Could you check a few things on this model? Use its own coordinates, in mm. A direction names the side the tool comes from. Coordinates: 2 decimals unless noted, no trailing zeros. Loops run counter-clockwise (first coordinate to the right, second up) from the corner with the lowest first, then second, coordinate; pieces in that order, holes last.
from build123d import *

# Parameters (mm, degrees)
SKETCH1_W                     = 42
SKETCH1_H                     = 20
BOSS_EXTRUDE1_DEPTH           = 40
CBORE_FOR_M5_SHCS1_AT_2_COUNT = 2
CBORE_FOR_M5_SHCS1_AT_2_PITCH = 20
SKETCH5_W                     = 42
SKETCH5_H                     = 20
BOSS_EXTRUDE2_DEPTH           = 6.5
SKETCH12_W                    = 21.9
SKETCH12_H                    = 10
BOSS_EXTRUDE3_DEPTH           = 46.5
CUT_EXTRUDE1_DEPTH            = 7.5
FILLET1_R                     = 1
CBORE_FOR_M3_SHCS2_AT_2_COUNT = 2
CBORE_FOR_M3_SHCS2_AT_2_PITCH = 20
CUT_EXTRUDE2_DEPTH            = 8


with BuildPart() as part:
    # Sketch1 → Boss-Extrude1 (new body)
    with BuildSketch(Plane(origin=(0, 0, 0), x_dir=(1, 0, 0), z_dir=(0, 1, 0))):
        Rectangle(SKETCH1_W, SKETCH1_H)
    extrude(amount=BOSS_EXTRUDE1_DEPTH)

    # Sketch4 → CBORE for M5 SHCS1 (revolve, cut)
    with BuildSketch(Plane(origin=(11, 30, 10), x_dir=(0, -1, 0), z_dir=(1, 0, 0))):
        Polygon((0, 0), (0, 20), (2.75, 20), (2.75, 5), (5, 5), (5, 0.020977491), (5.025, 0), align=None)
    cbore_for_m5_shcs1 = revolve(axis=Axis((11, 30, 16.35), (0, 0, -1)), mode=Mode.SUBTRACT)

    # CBORE for M5 SHCS1 at 2: CBORE for M5 SHCS1 ×2
    with Locations(*[(0, -i * CBORE_FOR_M5_SHCS1_AT_2_PITCH, 0) for i in range(1, CBORE_FOR_M5_SHCS1_AT_2_COUNT)]):
        add(cbore_for_m5_shcs1, mode=Mode.SUBTRACT)

    # Sketch5 → Boss-Extrude2 (add)
    with BuildSketch(Plane(origin=(0, 40, 0), x_dir=(1, 0, 0), z_dir=(0, 1, 0))):
        Rectangle(SKETCH5_W, SKETCH5_H)
    extrude(amount=BOSS_EXTRUDE2_DEPTH)

    # Sketch12 → Boss-Extrude3 (add)
    with BuildSketch(Plane(origin=(0, 46.5, 0), x_dir=(1, 0, 0), z_dir=(0, 1, 0))):
        with Locations((-10.05, 15)):
            Rectangle(SKETCH12_W, SKETCH12_H)
    extrude(amount=-BOSS_EXTRUDE3_DEPTH)

    # Sketch6 → Cut-Extrude1 (cut)
    with BuildSketch(Plane(origin=(0, 46.5, 0), x_dir=(1, 0, 0), z_dir=(0, 1, 0))):
        Polygon((-16.51, 20), (-16.51, -5), (-8.05, -5), (-8.05, 16), (-14.71, 16), (-14.71, 20), align=None)
    extrude(amount=-CUT_EXTRUDE1_DEPTH, mode=Mode.SUBTRACT)

    # Fillet1
    fillet1_edges = [part.edges().sort_by_distance(p)[0] for p in [
        (0.9, 23.25, -20),
        (-21, 23.25, -20),
        (21, 23.25, -10),
        (21, 23.25, 10),
        (-21, 23.25, 10),
    ]]
    fillet(fillet1_edges, radius=FILLET1_R)

    # Sketch11 → CBORE for M3 SHCS1 (revolve, cut)
    with BuildSketch(Plane(origin=(-11.48, 42.5, 10), x_dir=(0, -1, 0), z_dir=(1, 0, 0))):
        Polygon((0, 0), (0, 6.021463052), (1.7, 5), (1.7, 3), (3.25, 3), (3.25, 0.020977491), (3.275, 0), align=None)
    revolve(axis=Axis((-11.48, 42.5, 16.35), (0, 0, -1)), mode=Mode.SUBTRACT)

    # Sketch16 → CBORE for M3 SHCS2 (revolve, cut)
    with BuildSketch(Plane(origin=(-3.575, 46.5, -15), x_dir=(0, 0, 1), z_dir=(1, 0, 0))):
        Polygon((0, 0), (0, 46.5), (1.7, 46.5), (1.7, 3), (3.25, 3), (3.25, 0.020977491), (3.275, 0), align=None)
    cbore_for_m3_shcs2 = revolve(axis=Axis((-3.575, 52.85, -15), (0, -1, 0)), mode=Mode.SUBTRACT)

    # CBORE for M3 SHCS2 at 2: CBORE for M3 SHCS2 ×2
    with Locations(*[(0, 0, i * CBORE_FOR_M3_SHCS2_AT_2_PITCH) for i in range(1, CBORE_FOR_M3_SHCS2_AT_2_COUNT)]):
        add(cbore_for_m3_shcs2, mode=Mode.SUBTRACT)

    # Sketch18 → Cut-Extrude2 (cut)
    with BuildSketch(Plane.XZ):
        Polygon((-0.475, 5), (-2.025, 7.684678752), (-5.125, 7.684678752), (-6.675, 5), (-5.125, 2.315321248), (-2.025, 2.315321248), align=None)
        Polygon((-0.475, -15), (-2.025, -12.315321248), (-5.125, -12.315321248), (-6.675, -15), (-5.125, -17.684678752), (-2.025, -17.684678752), align=None)
    extrude(amount=-CUT_EXTRUDE2_DEPTH, mode=Mode.SUBTRACT)


solid = part.part
1) For faces 4 (the flat face through (-1.26, 3.94, 3.64)), 5 (the cylindrical face through (-11.55, 44.2, 6.01)), 6 (the flat face through (-14.71, 43, -18)), 7 (the cylindrical face through (-1.6, 45.01, -17.58)), which set-ups out of +Z, -Z, +X, -X, +Y, -Y let a thin tool reach every point of the face, with its end or its side?
2) Imagine slicing it at A-A on y = 30. List the corners of the cut face in (x, z) for me (3 decimals), plus the area to 3 significant figures.
3) Imagine slicing it at D-D on y = 42. State how many separate pieces and enclosed holes the cut face has, plus the area to 3 significant figures.
4) Imagine slicing it at C-C on z = -6.5. List the corners of the cut face in (x, y) for me.
5) Will these pins go through, and if not, where does the flat tip stop? pin 1 (2.5 mm diameter, centred on x = -3.575, z = -15, fed in from -Y); pin 2 (7 mm diameter, centred on y = 34, z = -14, fed in from +X); pin 3 (2.5 mm diameter, centred on x = -13.5, z = -5.5, fed in from +Y); pin 4 (7 mm diameter, centred on x = -10, y = 44, fed in from +Z).
6) Imagine slicing it at B-B on x = 11. List the corners of the cut face in (y, z) for me (3 decimals).
7) If I drill on L1, parallel to Y at x = 11, z = 0.25; L2, parallel to Y at x = 11, z = 8.25; L3, parallel to X at y = 31, z = -15 (3 decimals), over which ranges is the centre line in solid material (lowest first)?
8) We'd pull the mould along Z, two halves only. Please class faces 1 (the flat face through (10, 23, -10)), 2 (the flat face through (-12, 39, -5)), 3 (the flat face through (0.9, 24, -14)): released by +Z, released by -Z, zero draft, split by the parting line, or undercut.
Solved:
1. face 4: -Y
1. face 5: +Z
1. face 6: -Z, +Y
1. face 7: +Y
2. outline: (-21, -19) arc R1 ccw to (-20, -20) - (-0.1, -20) arc R1 ccw to (0.9, -19) - (0.9, -10) - (8.25, -10) - (8.25, 5) - (6, 5) - (6, 9.979) - (5.975, 10) - (-20, 10) arc R1 ccw to (-21, 9) - close; (13.75, -10) - (20, -10) arc R1 ccw to (21, -9) - (21, 9) arc R1 ccw to (20, 10) - (16.025, 10) - (16, 9.979) - (16, 5) - (13.75, 5) - close; hole circle Ø3.4 at (-3.575, -15); hole circle Ø3.4 at (-3.575, 5)
2. area: 907 mm2
3. separate pieces: 2
3. enclosed holes: 2
3. area: 829 mm2
4. outline: (-21, 0) - (21, 0) - (21, 46.5) - (-8.05, 46.5) - (-8.05, 39) - (-16.51, 39) - (-16.51, 46.5) - (-21, 46.5) - close; hole circle Ø5.5 at (11, 10); hole circle Ø5.5 at (11, 30)
5. pin 1: passes through
5. pin 2: stops at x = 0.9
5. pin 3: stops at y = 39
5. pin 4: stops at z = 10
6. outline: (0, -10) - (7.25, -10) - (7.25, 5) - (5, 5) - (5, 9.979) - (4.975, 10) - (0, 10) - close; (12.75, -10) - (27.25, -10) - (27.25, 5) - (25, 5) - (25, 9.979) - (24.975, 10) - (15.025, 10) - (15, 9.979) - (15, 5) - (12.75, 5) - close; (32.75, -10) - (46.5, -10) - (46.5, 10) - (35.025, 10) - (35, 9.979) - (35, 5) - (32.75, 5) - close
7. L1: y = 0 to 7.25, 12.75 to 27.25, 32.75 to 46.5
7. L2: y = 0 to 5, 15 to 25, 35 to 46.5
7. L3: x = -21 to -5.275, -1.875 to 0.9
8. face 1: released by -Z
8. face 2: undercut
8. face 3: zero draft
